Answer from the drawing. Dimensions are ordinates in mm from the lowest x, y and z of the part. Round coordinates to 2 decimals unless told otherwise and drop trailing zeros. Write each loop counter-clockwise with the first axis right and the second up, starting at its lowest first coordinate (ties: lowest second). Pieces come first, ordered by that corner, then holes. Notation, with made-up numbers: M 8,55.5 L 44,55.5 A20 ccw 44,67.5 Z; hole C 5,-19 d6. An arc over 180 degrees is marked long. One line per item, written item: value. Start each with the question number.
(1) Consider probe 1 along Y at (x, z) = (20, 3.8); probe 2 along Y at (x, z) = (18, 2.6); probe 3 along X at (y, z) = (11.5, 2.4). Determine where each line is inside the solid, lowest interval first.
(2) Section B-B (y = 60) is taken. Determine the outline of the cut face in (x, z), plus the area to 3 significant figures.
(3) Given P1, Ø8, axis at x = 20, y = 10, coming from the +Z side; P2, Ø2, axis at x = 25.5, y = 88.5, coming from the -Z side, each flat-ended and moving along its own axis, determine where each tip first touches the part or whether it passes through.
(4) For a pull along X with two mould halves and no side action, classify the marked faces 1, 2 and 3 as released by +X, released by -X, zero draft, split by the parting line, or undercut.
(5) Section D-D (x = 36) is taken. Determine the outline of the cut face in (y, z), plus the area to 3 significant figures.
(6) Section A-A (x = 20) is taken. Determine the outline of the cut face in (y, z).
(7) Section C-C (z = 3) is taken. Determine the outline of the cut face in (x, y), plus the area to 3 significant figures.
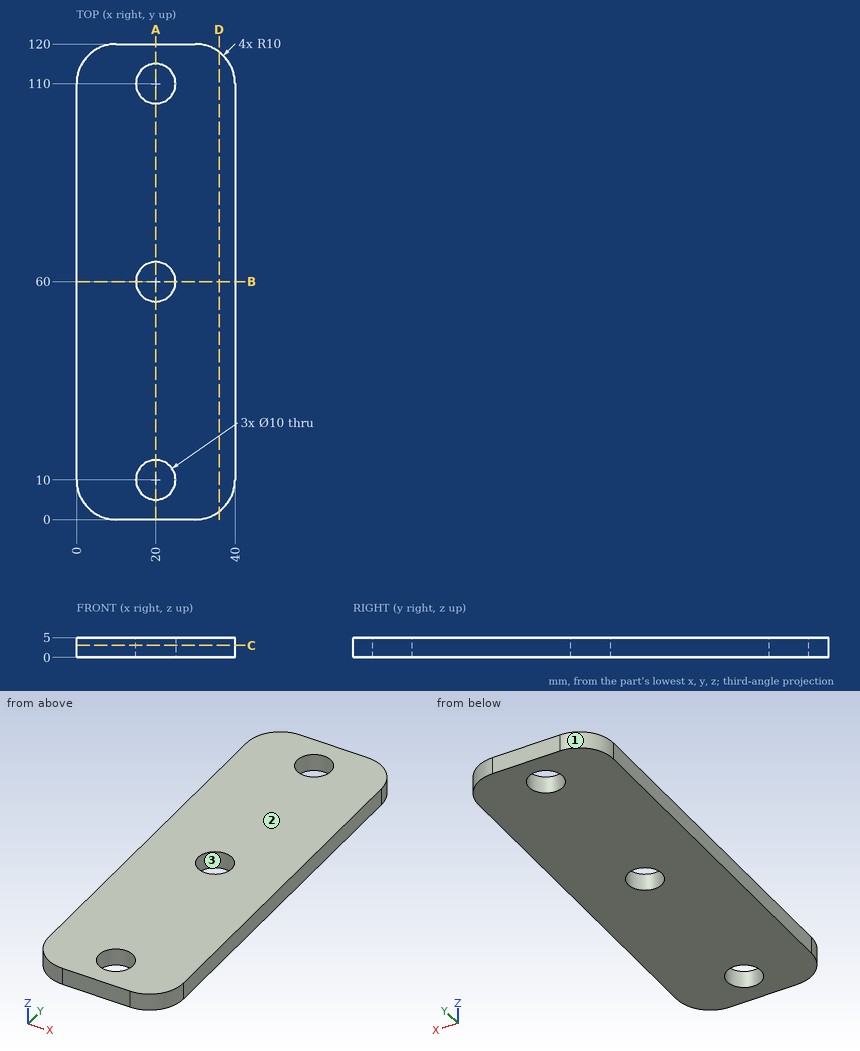
Recorded:
1. probe 1: y = 0 to 5, 15 to 55, 65 to 105, 115 to 120
1. probe 2: y = 0 to 5.42, 14.58 to 55.42, 64.58 to 105.42, 114.58 to 120
1. probe 3: x = 0 to 15.23, 24.77 to 40
2. outline: M 0,0 L 15,0 L 15,5 L 0,5 Z; M 25,0 L 40,0 L 40,5 L 25,5 Z
2. area: 150 mm2
3. P1: passes through
3. P2: stops at z = 0
4. face 1: released by -X
4. face 2: zero draft
4. face 3: undercut
5. outline: M 2,0 L 118,0 L 118,5 L 2,5 Z
5. area: 580 mm2
6. outline: M 0,0 L 5,0 L 5,5 L 0,5 Z; M 15,0 L 55,0 L 55,5 L 15,5 Z; M 65,0 L 105,0 L 105,5 L 65,5 Z; M 115,0 L 120,0 L 120,5 L 115,5 Z
7. outline: M 0,10 A10 ccw 10,0 L 30,0 A10 ccw 40,10 L 40,110 A10 ccw 30,120 L 10,120 A10 ccw 0,110 Z; hole C 20,10 d10; hole C 20,60 d10; hole C 20,110 d10
7. area: 4,480 mm2
